```python
from build123d import *

# Parameters (mm, degrees)
SKETCH_R      = 8
PAD_DEPTH     = 5
PAD001_DEPTH  = 20
CHAMFER_SIZE  = 1
SKETCH002_R   = 10
SKETCH002_R_2 = 6
PAD002_DEPTH  = 2


with BuildPart() as part:
    # Sketch → Pad (new body)
    with BuildSketch(Plane.XY):
        with BuildLine():
            ThreePointArc((-2.4, -9.707729), (10, 0), (-2.4, 9.707729))
            Line((-25.96, 3.883092), (-2.4, 9.707729))
            ThreePointArc((-25.96, 3.883092), (-29, 0), (-25.96, -3.883092))
            Line((-2.4, -9.707729), (-25.96, -3.883092))
        make_face()
        Circle(SKETCH_R, mode=Mode.SUBTRACT)
    extrude(amount=PAD_DEPTH)

    # Sketch001 (on Face7 of Pad) → Pad001 (join)
    with BuildSketch(Plane.XY.offset(5)):
        with BuildLine():
            ThreePointArc((-25.96, 3.883092), (-29, 0), (-25.96, -3.883092))
            Line((-21, -5.109331), (-25.96, -3.883092))
            Line((-21, -5.109331), (-21, 5.109331))
            Line((-21, 5.109331), (-25.96, 3.883092))
        make_face()
    extrude(amount=PAD001_DEPTH)

    # Chamfer
    chamfer_edges = [part.edges().sort_by_distance(p)[0] for p in [
        (-8, 0, 5),
    ]]
    chamfer(chamfer_edges, length=CHAMFER_SIZE)

    # Sketch002 (on Face9 of Chamfer) → Pad002 (join)
    with BuildSketch(Plane(origin=(0, 0, 0), x_dir=(1, 0, 0), z_dir=(0, 0, -1))):
        Circle(SKETCH002_R)
        Circle(SKETCH002_R_2, mode=Mode.SUBTRACT)
    extrude(amount=PAD002_DEPTH)


solid = part.part
```
Geometry check sheet. Reference: the model listing, model coordinates, mm. A direction names the side the tool comes from. Give positions to 0.01 mm unless a question says otherwise; leave off trailing zeros. Write each loop counter-clockwise with the first axis right and the second up, starting at its lowest first coordinate (ties: lowest second). Pieces come first, ordered by that corner, then holes. Notation, with made-up numbers: (73, 73.25) -> (107, 73.25) arc R17 ccw to (107, 88.25) -> close; hole circle Ø8 at (75, 11.5). An arc over 180 degrees is marked (long way). One line per question, with ' | ' between items.
Item 1: Scan lines: line 1 along Y through (x, z) = (0, -0.8); line 2 along Y through (x, z) = (0, 1.85). Record each from-to range of solid material in increasing order.
Determined:
line 1: -10 to -6, 6 to 10 | line 2: -10 to -8, 8 to 10
Item 2: Draft check along Y on faces 1 (the flat face through (-23.445, 4.505, 14.86)), 2 (the cylindrical face through (-1.73, -7.81, 1.97)), 3 (the flat face through (-24, 0, 25)). Enter one of: released by +Y, released by -Y, zero draft, split by the parting line, or undercut.
Determined:
face 1: released by +Y | face 2: undercut | face 3: zero draft
Item 3: Sectioned sample at B-B, the plane y = 0. Record the boundary of the cut face in (x, z).
Determined:
outline: (-29, 0) -> (-10, 0) -> (-10, -2) -> (-6, -2) -> (-6, 0) -> (-8, 0) -> (-8, 4) -> (-9, 5) -> (-21, 5) -> (-21, 25) -> (-29, 25) -> close; (6, -2) -> (10, -2) -> (10, 5) -> (9, 5) -> (8, 4) -> (8, 0) -> (6, 0) -> close
Item 4: Sectioned sample at D-D, the plane x = -25. Record the boundary of the cut face in (y, z).
Determined:
outline: (-4.12, 0) -> (4.12, 0) -> (4.12, 25) -> (-4.12, 25) -> close
Item 5: Access from +Z, -Z, +X, -X, +Y, -Y to the whole of each face (thin tool, end or side, straight path). Record for faces 4 (the flat face through (0, 7, -2)), 5 (the flat face through (-2, -6, 0)), 6 (the flat face through (-21, 0, 15)).
Determined:
face 4: -Z, +X, -X, +Y, -Y | face 5: +Z | face 6: +Z, +X, +Y, -Y
Item 6: Sectioned sample at C-C, the plane z = 2.25. Record the boundary of the cut face in (x, y).
Determined:
outline: (-25.96, -3.88) -> (-2.4, -9.71) arc R10 ccw (long way) to (-2.4, 9.71) -> (-25.96, 3.88) arc R4 ccw to start; hole circle Ø16 at (0, 0)
Item 7: Depth check by flat-ended pin: pin 1 (5 mm diameter, centred on y = -0.5, z = 13.5, fed in from +X); pin 2 (1.5 mm diameter, centred on x = -10, y = -4.5, fed in from +Z); pin 3 (6 mm diameter, centred on x = -23, z = 6.5, fed in from +Y). Enter the tip coordinate at first touch or a pass-through.
Determined:
pin 1: x = -21 | pin 2: z = 5 | pin 3: y = 5.26
Item 8: Sectioned sample at A-A, the plane x = 0. Record the boundary of the cut face in (y, z).
Determined:
outline: (-10, -2) -> (-6, -2) -> (-6, 0) -> (-8, 0) -> (-8, 4) -> (-9, 5) -> (-10, 5) -> close; (6, -2) -> (10, -2) -> (10, 5) -> (9, 5) -> (8, 4) -> (8, 0) -> (6, 0) -> close
